Read the model definition and answer for the solid it produces. Units are mm, in the model's axes. Give positions to 0.01 mm unless a question says otherwise; leave off trailing zeros. Write each loop counter-clockwise with the first axis right and the second up, starting at its lowest first coordinate (ties: lowest second). Pieces come first, ordered by that corner, then holes. Notation, with made-up numbers: (19.5, 34.25) - (47.5, 34.25) arc R33 ccw to (47.5, 62.25) - close; hole circle Ø5 at (65.5, -24.5). An arc over 180 degrees is marked (long way). Answer as CSV lines item,"result".
```python
from build123d import *

# Parameters (mm, degrees)
SKETCH1_W           = 463.55
SKETCH1_H           = 814.3875
BOSS_EXTRUDE1_DEPTH = 3.175
FILLET1_R           = 3.175
CUT_EXTRUDE2_REACH  = 939.078
SKETCH3_W           = 31.75
SKETCH3_H           = 31.75
FILLET2_R           = 3.175
FILLET3_R           = 3.175
FILLET4_R           = 3.175


with BuildPart() as part:
    # Sketch1 → Boss-Extrude1 (new body)
    with BuildSketch(Plane(origin=(0, 0, 0), x_dir=(0, 0, -1), z_dir=(1, 0, 0))):
        with Locations((231.775, 407.19375)):
            Rectangle(SKETCH1_W, SKETCH1_H)
    extrude(amount=BOSS_EXTRUDE1_DEPTH)

    # Fillet1
    fillet1_edges = [part.edges().sort_by_distance(p)[0] for p in [
        (1.5875, 814.3875, 0),
        (1.5875, 814.3875, -463.55),
        (1.5875, 0, -463.55),
        (1.5875, 0, 0),
    ]]
    fillet(fillet1_edges, radius=FILLET1_R)

    # Sketch3 → Cut-Extrude2 (cut, up to next)
    with BuildSketch(Plane(origin=(3.175, 0, 0), x_dir=(0, 0, -1), z_dir=(1, 0, 0)), mode=Mode.PRIVATE) as cut_extrude2_sk1:
        with Locations((15.875, 754.0625)):
            Rectangle(SKETCH3_W, SKETCH3_H)
    cut_extrude2_tool1 = extrude(cut_extrude2_sk1.sketch, amount=-CUT_EXTRUDE2_REACH, mode=Mode.PRIVATE) & part.part
    # Sketch3 → Cut-Extrude2 (cut, up to next)
    with BuildSketch(Plane(origin=(3.175, 0, 0), x_dir=(0, 0, -1), z_dir=(1, 0, 0)), mode=Mode.PRIVATE) as cut_extrude2_sk2:
        with Locations((447.675, 754.0625)):
            Rectangle(SKETCH3_W, SKETCH3_H)
    cut_extrude2_tool2 = extrude(cut_extrude2_sk2.sketch, amount=-CUT_EXTRUDE2_REACH, mode=Mode.PRIVATE) & part.part
    # Sketch3 → Cut-Extrude2 (cut, up to next)
    with BuildSketch(Plane(origin=(3.175, 0, 0), x_dir=(0, 0, -1), z_dir=(1, 0, 0)), mode=Mode.PRIVATE) as cut_extrude2_sk3:
        with Locations((447.675, 15.875)):
            Rectangle(SKETCH3_W, SKETCH3_H)
    cut_extrude2_tool3 = extrude(cut_extrude2_sk3.sketch, amount=-CUT_EXTRUDE2_REACH, mode=Mode.PRIVATE) & part.part
    # Sketch3 → Cut-Extrude2 (cut, up to next)
    with BuildSketch(Plane(origin=(3.175, 0, 0), x_dir=(0, 0, -1), z_dir=(1, 0, 0)), mode=Mode.PRIVATE) as cut_extrude2_sk4:
        with Locations((15.875, 15.875)):
            Rectangle(SKETCH3_W, SKETCH3_H)
    cut_extrude2_tool4 = extrude(cut_extrude2_sk4.sketch, amount=-CUT_EXTRUDE2_REACH, mode=Mode.PRIVATE) & part.part
    add(cut_extrude2_tool1.solids().sort_by_distance((3.175, 754.0625, -15.875))[0], mode=Mode.SUBTRACT)
    add(cut_extrude2_tool2.solids().sort_by_distance((3.175, 754.0625, -447.675))[0], mode=Mode.SUBTRACT)
    add(cut_extrude2_tool3.solids().sort_by_distance((3.175, 15.875, -447.675))[0], mode=Mode.SUBTRACT)
    add(cut_extrude2_tool4.solids().sort_by_distance((3.175, 15.875, -15.875))[0], mode=Mode.SUBTRACT)

    # Fillet2
    fillet2_edges = [part.edges().sort_by_distance(p)[0] for p in [
        (1.5875, 738.1875, 0),
        (1.5875, 769.9375, 0),
        (1.5875, 769.9375, -31.75),
        (1.5875, 738.1875, -31.75),
    ]]
    fillet(fillet2_edges, radius=FILLET2_R)

    # Fillet3
    fillet3_edges = [part.edges().sort_by_distance(p)[0] for p in [
        (1.5875, 769.9375, -431.8),
        (1.5875, 769.9375, -463.55),
        (1.5875, 738.1875, -463.55),
        (1.5875, 738.1875, -431.8),
    ]]
    fillet(fillet3_edges, radius=FILLET3_R)

    # Fillet4
    fillet4_edges = [part.edges().sort_by_distance(p)[0] for p in [
        (1.5875, 31.75, 0),
        (1.5875, 31.75, -31.75),
        (1.5875, 0, -31.75),
        (1.5875, 0, -431.8),
        (1.5875, 31.75, -431.8),
        (1.5875, 31.75, -463.55),
    ]]
    fillet(fillet4_edges, radius=FILLET4_R)


solid = part.part
```
(1) A cutting plane is placed at A-A (y = 752.5). Write down the section's boundary in (x, z) (3 decimals), and give its area (3 significant figures).
Worked out:
outline,"(0, -431.8) - (3.175, -431.8) - (3.175, -31.75) - (0, -31.75) - close"
area,"1,270 mm^2"
(2) Each of these flat-tipped pins is pushed along its axis until it touches: P1, Ø1.6, axis at x = 2, y = 749.5, coming from the -Z side; P2, Ø1.6, axis at x = 1.5, y = 19.5, coming from the +Z side; P3, Ø1.6, axis at x = 2, z = -444, coming from the -Y side. Where does it stop, or does it pass through?
Worked out:
P1,"stops at z = -431.8"
P2,"stops at z = -31.75"
P3,"stops at y = 31.75"
(3) The mould has two halves that part along X. Classify faces 1 (the flat face through (3.175, 413, -229)), 2 (the flat face through (0, 413, -229)): +X half, -X half, draft (parallel to the pull), parting line (faces both ways), or undercut.
Worked out:
face 1,"+X half"
face 2,"-X half"
(4) Find the intervals of material crossed by L1, parallel to Y at x = 2.6, z = -434; L2, parallel to Z at x = 2.45, y = 756; L3, parallel to Z at x = 2.45, y = 33, in increasing order.
Worked out:
L1,"y = 31.6 to 738.34, 769.78 to 814.39"
L2,"z = -431.8 to -31.75"
L3,"z = -462.9 to -0.65"
